Build history of the part. All positions in model axes, mm. Face numbers are marked on the shaded views. A direction names the side the tool comes from. Give positions to 0.01 mm unless a question says otherwise; leave off trailing zeros. Order: outer loops, then holes, each group sorted by start corner. A loop starts at its lowest first (then second) coordinate and runs counter-clockwise, first axis right, second up. Notation, with made-up numbers: (48.25, 27.25) -> (60.25, 27.25) arc R29 cw to (60.25, 49.25) -> close; hole circle Ø6 at (44.25, 27.5). An arc over 180 degrees is marked (long way). One line per question, with ' | ' between items. Start each with the question number.
(1) Drill centre lines: L1, parallel to Z at x = 6.5, y = 0.15 (3 decimals); L2, parallel to Z at x = 2, y = 1.5 (3 decimals); L3, parallel to X at y = 0.35, z = -0.75 (3 decimals). Where is each one in solid material? Low to high. Write a range as from..to.
(2) Pin check, flat tips, straight feed: pin 1 Ø2 at (x, z) = (2.5, -4.5) entering from -Y (3 decimals); pin 2 Ø4 at (x, z) = (4.5, -8) entering from +Y. Stop position of each tip, or through.
(3) Cut at A-A (y = 1.1). Give the cut face in (x, z) (3 decimals).
(4) Cut at D-D (x = 4.5). Give the cut face in (y, z) (3 decimals), then the cut area to 3 significant figures.
(5) Cut at B-B (z = -9.25). Give the cut face in (x, y) (3 decimals).
(6) Cut at C-C (x = 11). Give the cut face in (y, z) (3 decimals).
(7) Pull direction Z, two halves, no side cores. Call the marked faces 3, 4, 5 and 6: +Z half, -Z half, draft (parallel to the pull), parting line (faces both ways), or undercut.
(8) Which spindle directions (+Z, -Z, +X, -X, +Y, -Y) get a long thin tool onto all of the face, cutting with end or side? Do the marked faces 1 and 2. Say none if no direction does.
from build123d import *

# Parameters (mm, degrees)
SKETCH1_W           = 12.7
SKETCH1_H           = 12.7
BOSS_EXTRUDE1_DEPTH = 2.54
FILLET1_R           = 0.635
SHELL1_START        = 0.635
SHELL1_OUTLINE_W    = 1.905
SHELL1_OUTLINE_H    = 11.43
SHELL1_DEPTH        = 11.43
SKETCH2_R           = 2.54
BOSS_EXTRUDE2_DEPTH = 1.905
BOSS_EXTRUDE3_DEPTH = 0.00254


# Read off the part's stored shape, not the designer's step: Shell1
with BuildPart() as part:
    # Sketch1 → Boss-Extrude1 (new body)
    with BuildSketch(Plane(origin=(0, 0, 0), x_dir=(1, 0, 0), z_dir=(0, 1, 0))):
        with Locations((6.35, 6.35)):
            Rectangle(SKETCH1_W, SKETCH1_H)
    extrude(amount=BOSS_EXTRUDE1_DEPTH)

    # Fillet1
    fillet1_edges = [part.edges().sort_by_distance(p)[0] for p in [
        (0, 1.27, -12.7),
        (12.7, 1.27, -12.7),
        (12.7, 1.27, 0),
        (0, 1.27, 0),
    ]]
    fillet(fillet1_edges, radius=FILLET1_R)

    # Shell1 outline → Shell1 (cut)
    with BuildSketch(Plane.YZ.offset(SHELL1_START)):
        with Locations((0.9525, -6.35)):
            Rectangle(SHELL1_OUTLINE_W, SHELL1_OUTLINE_H)
    extrude(amount=SHELL1_DEPTH, mode=Mode.SUBTRACT)

    # Sketch2 → Boss-Extrude2 (add)
    with BuildSketch(Plane(origin=(0, 1.905, 0), x_dir=(-1, 0, 0), z_dir=(0, -1, 0))):
        with Locations(Location((-6.35, 6.35, 0), (0, 0, 270))):
            Circle(SKETCH2_R)
    extrude(amount=BOSS_EXTRUDE2_DEPTH)

    # Sketch3 → Boss-Extrude3 (add)
    with BuildSketch(Plane(origin=(0, 2.54, 0), x_dir=(1, 0, 0), z_dir=(0, 1, 0))):
        Polygon((7.012679487, 9.564076923), (6.687038462, 9.564076923), (6.564923077, 10.622410256), (7.134794872, 10.622410256), align=None)
        Polygon((6.117166667, 9.564076923), (5.791525641, 9.564076923), (5.669410256, 10.622410256), (6.239282051, 10.622410256), align=None)
        Polygon((6.493282051, 5.246076923), (6.167641026, 5.246076923), (6.045525641, 6.304410256), (6.615397436, 6.304410256), align=None)
    extrude(amount=BOSS_EXTRUDE3_DEPTH)


solid = part.part
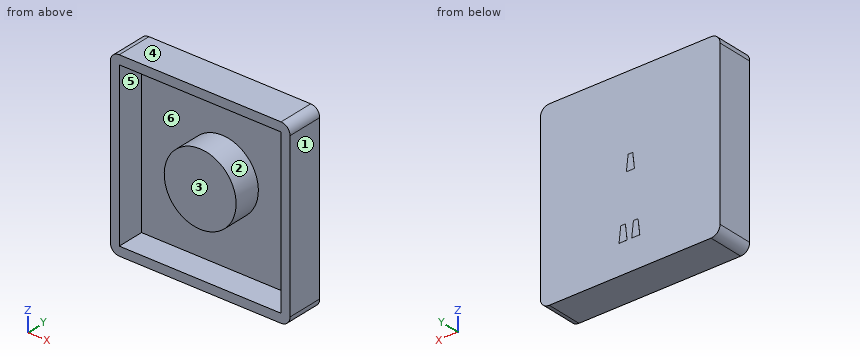
Result set:
1) L1: z = -12.7..-12.065, -8.886..-3.814, -0.635..0 | L2: z = -12.7..-12.065, -0.635..0 | L3: x = 0..0.635, 12.065..12.7
2) pin 1: stops at y = 1.905 | pin 2: stops at y = 2.54
3) outline: (0, -12.065) arc R0.635 ccw to (0.635, -12.7) -> (12.065, -12.7) arc R0.635 ccw to (12.7, -12.065) -> (12.7, -0.635) arc R0.635 ccw to (12.065, 0) -> (0.635, 0) arc R0.635 ccw to (0, -0.635) -> close; circle Ø5.08 at (6.35, -6.35); hole (0.635, -12.065) -> (12.065, -12.065) -> (12.065, -0.635) -> (0.635, -0.635) -> close
4) outline: (0, -12.7) -> (2.54, -12.7) -> (2.54, 0) -> (0, 0) -> (0, -0.635) -> (1.905, -0.635) -> (1.905, -4.61) -> (0, -4.61) -> (0, -8.09) -> (1.905, -8.09) -> (1.905, -12.065) -> (0, -12.065) -> close | area: 17.1 mm2
5) outline: (0, 0) -> (0.635, 0) -> (0.635, 1.905) -> (12.065, 1.905) -> (12.065, 0) -> (12.7, 0) -> (12.7, 2.54) -> (0, 2.54) -> close
6) outline: (0, -12.7) -> (2.54, -12.7) -> (2.54, 0) -> (0, 0) -> (0, -0.635) -> (1.905, -0.635) -> (1.905, -12.065) -> (0, -12.065) -> close
7) face 3: draft | face 4: +Z half | face 5: undercut | face 6: undercut
8) face 1: +Z, -Z, +X, +Y, -Y | face 2: -Y
